```python
from build123d import *

# Parameters (mm, degrees)
SKIZZE1_R                       = 5
AUFSATZ_LINEAR_AUSTRAGEN1_DEPTH = 90
SKIZZE2_R                       = 5
AUFSATZ_LINEAR_AUSTRAGEN2_DEPTH = 30
SKIZZE3_W                       = 92
SKIZZE3_H                       = 100
SCHNITT_LINEAR_AUSTRAGEN1_DEPTH = 295.78805946


with BuildPart() as part:
    # Skizze1 → Aufsatz-Linear austragen1 (new body)
    with BuildSketch(Plane.XY):
        with BuildLine():
            Line((50, 0), (50, 200))
            ThreePointArc((50, 200), (0, 250), (-50, 200))
            Line((-50, 200), (-50, 0))
            ThreePointArc((-50, 0), (0, -50), (50, 0))
        make_face()
        with Locations(Location((0, 200, 0), (0, 0, 180))):
            Circle(SKIZZE1_R, mode=Mode.SUBTRACT)
        with Locations(Location((0, 0, 0), (0, 0, 180))):
            Circle(SKIZZE1_R, mode=Mode.SUBTRACT)
    extrude(amount=AUFSATZ_LINEAR_AUSTRAGEN1_DEPTH)

    # Skizze2 → Aufsatz-Linear austragen2 (add)
    # profile 1 of 2: a face of its own
    with BuildSketch(Plane.XY.offset(90)):
        with BuildLine():
            ThreePointArc((50, 200), (0, 250), (-50, 200))
            ThreePointArc((-50, 200), (0, 150), (50, 200))
        make_face()
        with Locations(Location((0, 200, 0), (0, 0, 180))):
            Circle(SKIZZE2_R, mode=Mode.SUBTRACT)
    # profile 2 of 2: a face of its own
    with BuildSketch(Plane.XY.offset(90)):
        with BuildLine():
            ThreePointArc((50, 200), (0, 150), (-50, 200))
            Line((-50, 200), (-50, 113.397459622))
            ThreePointArc((-50, 113.397459622), (0, 100), (50, 113.397459622))
            Line((50, 113.397459622), (50, 200))
        make_face()
    aufsatz_linear_austragen2 = extrude(amount=AUFSATZ_LINEAR_AUSTRAGEN2_DEPTH)

    # Spiegeln1: Aufsatz-Linear austragen2 across plane
    add(aufsatz_linear_austragen2.mirror(Plane(origin=(0, 0, 45), x_dir=(1, 0, 0), z_dir=(0, 0, -1))))

    # Skizze3 → Schnitt-Linear austragen1 (cut, through all)
    with BuildSketch(Plane.ZY.offset(50)):
        with Locations((45, 200)):
            Rectangle(SKIZZE3_W, SKIZZE3_H)
    extrude(amount=-SCHNITT_LINEAR_AUSTRAGEN1_DEPTH, mode=Mode.SUBTRACT)


solid = part.part
```
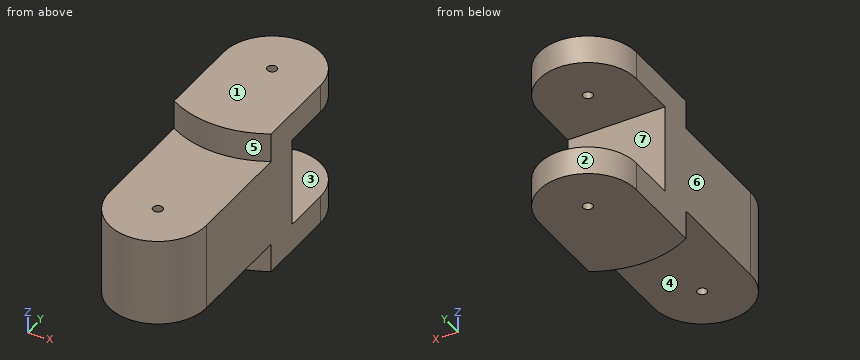
The listing builds one solid part. Answer for the finished solid, in the listing's coordinates (mm). Face numbers are marked on the shaded views. A direction names the side the tool comes from. Give positions to 0.01 mm unless a question says otherwise; leave off trailing zeros. Loops run counter-clockwise (first coordinate to the right, second up) from the corner with the lowest first, then second, coordinate; pieces in that order, holes last. Notation, with made-up numbers: (-1, 17.25) - (56, 17.25) arc R29 ccw to (56, 42.25) - close; hole circle Ø3 at (30, -31). An arc over 180 degrees is marked (long way). Answer as CSV lines item,"result". Start each with the question number.
Item 1: A cutting plane is placed at C-C on z = 4.5. Determine the outline of the cut face in (x, y).
Item 2: Each of these flat-tipped pins is pushed along its axis until it touches: pin 1 (4 mm diameter, centred on x = 32, z = 76, fed in from +Y); pin 2 (9 mm diameter, centred on x = 0, y = 200, fed in from -Z); pin 3 (8 mm diameter, centred on x = -30, y = 58.5, fed in from +Z); pin 4 (6 mm diameter, centred on x = -4, y = 45.5, fed in from -Z). Where does it stop, or does it pass through?
Item 3: A cutting plane is placed at A-A on y = 181.5. Determine the outline of the cut face in (x, z), then the cut area to 3 significant figures.
Item 4: A cutting plane is placed at B-B on x = 0. Determine the outline of the cut face in (y, z).
Item 5: For the marked faces 5, 6 and 7, determine the directions among +Z, -Z, +X, -X, +Y, -Y from which every point of the face is accessible in a straight line to the end or side of a thin tool.
Item 6: The mould has two halves that part along Z. Classify the marked faces 1, 2, 3 and 4: +Z half, -Z half, draft (parallel to the pull), parting line (faces both ways), or undercut.
Item 7: Find the intervals of material crossed by line 1 (Y direction, x = 0, z = 43); line 2 (Z direction, x = 7, y = 189.5); line 3 (X direction, y = 200, z = 100.75), in increasing order. Write a range as from..to.
Item 8: A cutting plane is placed at D-D on x = -24. Determine the outline of the cut face in (y, z).
Found:
1,outline,"(-50, 0) arc R50 ccw to (50, 0) - (50, 150) - (-50, 150) - close; hole circle Ø10 at (0, 0)"
2,pin 1,"stops at y = 150"
2,pin 2,"passes through"
2,pin 3,"stops at z = 90"
2,pin 4,"stops at z = 0"
3,outline,"(-50, -30) - (50, -30) - (50, -1) - (-50, -1) - close; (-50, 91) - (50, 91) - (50, 120) - (-50, 120) - close"
3,area,"5,800 mm^2"
4,outline,"(-50, 0) - (-5, 0) - (-5, 90) - (-50, 90) - close; (5, 0) - (100, 0) - (100, -30) - (195, -30) - (195, -1) - (150, -1) - (150, 91) - (195, 91) - (195, 120) - (100, 120) - (100, 90) - (5, 90) - close; (205, -30) - (250, -30) - (250, -1) - (205, -1) - close; (205, 91) - (250, 91) - (250, 120) - (205, 120) - close"
5,face 5,"+Z, -Y"
5,face 6,"+Z, -Z, -X, +Y, -Y"
5,face 7,"+X, -X, +Y"
6,face 1,"+Z half"
6,face 2,"draft"
6,face 3,"undercut"
6,face 4,"-Z half"
7,line 1,"y = -50..-5, 5..150"
7,line 2,"z = -30..-1, 91..120"
7,line 3,"x = -50..-5, 5..50"
8,outline,"(-43.86, 0) - (102.92, 0) - (102.92, -30) - (243.86, -30) - (243.86, -1) - (150, -1) - (150, 91) - (243.86, 91) - (243.86, 120) - (102.92, 120) - (102.92, 90) - (-43.86, 90) - close"
